Print and shaded views of the part. All mm, measured from the part's lowest x, y and z. A direction names the side the tool comes from. Coordinates: 2 decimals unless noted, no trailing zeros. Order: outer loops, then holes, each group sorted by start corner. A loop starts at its lowest first (then second) coordinate and runs counter-clockwise, first axis right, second up.
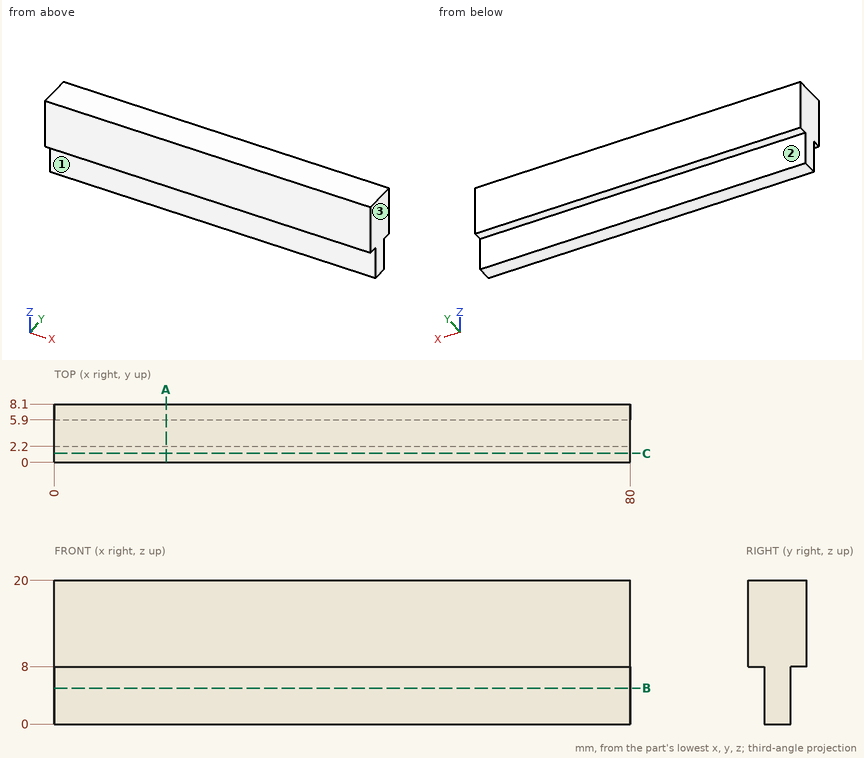
Q1. Which spindle directions (+Z, -Z, +X, -X, +Y, -Y) get a long thin tool onto all of the face, cutting with end or side? Do the marked faces 1, 2 and 3. Say none if no direction does.
Established:
face 1: -Z, +X, -X, -Y
face 2: -Z, +X, -X, +Y
face 3: +Z, -Z, +X, +Y, -Y
Q2. Drop flat-ended pins along their axis: P1, Ø6.5, axis at x = 37, z = 4.5, coming from the -Y side; P2, Ø1, axis at x = 52, y = 6, coming from the -Z side; P3, Ø1.1, axis at x = 39, y = 1, coming from the -Z side. Give the stop position or say it passes through.
Established:
P1: stops at y = 2.2
P2: stops at z = 0
P3: stops at z = 8
Q3. Cut at C-C, the plane y = 1.25. List the corners of the cut face in (x, z).
Established:
outline: (0, 8) - (80, 8) - (80, 20) - (0, 20) - close
Q4. Cut at A-A, the plane x = 15.5. List the corners of the cut face in (y, z), plus the area to 3 significant figures.
Established:
outline: (0, 8) - (2.2, 8) - (2.2, 0) - (5.9, 0) - (5.9, 8) - (8.1, 8) - (8.1, 20) - (0, 20) - close
area: 127 mm2
Q5. Probe line 1 (Z direction, x = 47, y = 1.75); line 2 (Y direction, x = 67.5, z = 7.25). List the from-to ranges inside material, lowest first.
Established:
line 1: z = 8 to 20
line 2: y = 2.2 to 5.9
Q6. Cut at B-B, the plane z = 5. List the corners of the cut face in (x, y).
Established:
outline: (0, 2.2) - (80, 2.2) - (80, 5.9) - (0, 5.9) - close
